from build123d import *

# Parameters (mm, degrees)
SKETCH_1_W                  = 104.137931034
SKETCH_1_H                  = 70
EXTRUDE_1_DEPTH             = 3
SKETCH_2_R                  = 1.75
CUT_EXTRUDE_1_DEPTH         = 10
PATTERN_LINEAR_1_COUNT      = 2
PATTERN_LINEAR_1_PITCH      = 60
PATTERN_LINEAR_1_COUNT_DIR2 = 2
PATTERN_LINEAR_1_PITCH_DIR2 = 40
CUT_EXTRUDE_2_DEPTH         = 4
SKETCH_4_R                  = 4
CUT_EXTRUDE_3_DEPTH         = 4
FILLET_1_R                  = 7


with BuildPart() as part:
    # Эскиз1 → Бобышка-Вытянуть1 (new body)
    with BuildSketch(Plane(origin=(0, 0, 0), x_dir=(1, 0, 0), z_dir=(0, 1, 0))):
        Rectangle(SKETCH_1_W, SKETCH_1_H)
    extrude(amount=EXTRUDE_1_DEPTH)

    # Эскиз2 → Вырез-Вытянуть1 (cut)
    with BuildSketch(Plane(origin=(0, 3, 0), x_dir=(1, 0, 0), z_dir=(0, 1, 0))):
        with Locations((-43.318965517, 26.25)):
            Circle(SKETCH_2_R)
    cut_extrude_1 = extrude(amount=-CUT_EXTRUDE_1_DEPTH, mode=Mode.SUBTRACT)

    # Линейный массив1: Cut-Extrude 1 2 × 2
    with Locations(*[(i * PATTERN_LINEAR_1_PITCH, 0, j * PATTERN_LINEAR_1_PITCH_DIR2) for i in range(PATTERN_LINEAR_1_COUNT) for j in range(PATTERN_LINEAR_1_COUNT_DIR2) if (i, j) != (0, 0)]):
        add(cut_extrude_1, mode=Mode.SUBTRACT)

    # Эскиз3 → Вырез-Вытянуть2 (cut, through all)
    with BuildSketch(Plane(origin=(0, 3, 0), x_dir=(1, 0, 0), z_dir=(0, 1, 0))):
        Polygon((-52.068965517, -22.5), (25.431034483, -22.5), (25.431034483, 35), (52.068965517, 35), (52.068965517, -35), (-52.068965517, -35), align=None)
    extrude(amount=-CUT_EXTRUDE_2_DEPTH, mode=Mode.SUBTRACT)

    # Эскиз4 → Вырез-Вытянуть3 (cut, through all)
    with BuildSketch(Plane(origin=(0, 3, 0), x_dir=(1, 0, 0), z_dir=(0, 1, 0))):
        with Locations((-27.568965517, 6.25)):
            Circle(SKETCH_4_R)
        with BuildLine():
            Line((-13.318965517, 8.5), (8.681034483, 8.5))
            ThreePointArc((8.681034483, 8.5), (10.931034483, 6.25), (8.681034483, 4))
            Line((8.681034483, 4), (-13.318965517, 4))
            ThreePointArc((-13.318965517, 4), (-15.568965517, 6.25), (-13.318965517, 8.5))
        make_face()
    extrude(amount=-CUT_EXTRUDE_3_DEPTH, mode=Mode.SUBTRACT)

    # Скругление1
    fillet_1_edges = [part.edges().sort_by_distance(p)[0] for p in [
        (-52.068965517, 1.5, 22.5),
        (25.431034483, 1.5, 22.5),
        (25.431034483, 1.5, -35),
        (-52.068965517, 1.5, -35),
    ]]
    fillet(fillet_1_edges, radius=FILLET_1_R)


solid = part.part
Work out the finished part from the listing and answer in its coordinate system (mm). A direction names the side the tool comes from. Round coordinates to 2 decimals unless told otherwise and drop trailing zeros. Write each loop counter-clockwise with the first axis right and the second up, starting at its lowest first coordinate (ties: lowest second). Pieces come first, ordered by that corner, then holes. Notation, with made-up numbers: (34, -14.5) -> (73, -14.5) arc R11 ccw to (73, 0.5) -> close; hole circle Ø9 at (60.25, -10). An arc over 180 degrees is marked (long way). Answer as CSV lines item,"result". Start each with the question number.
(1) The part is cut by section D-D, the plane z = -6.25. Give the vertices of the cut face in (x, y), then the cut area to 3 significant figures.
(2) The part is cut by section C-C, the plane y = 0.45. Give the vertices of the cut face in (x, z), then the cut area to 3 significant figures.
(3) Find the intervals of material crossed by probe 1 along X at (y, z) = (1.2, 13.75); probe 2 along X at (y, z) = (1.85, -6.25); probe 3 along Z at (x, y) = (-3, 0.35), in increasing order.
(4) The part is cut by section A-A, the plane z = 13.75. Give the vertices of the cut face in (x, y).
(5) The mould has two halves that part along X. Classify faces 1 (the flat face through (-14, 1, -35)), 2 (the cylindrical face through (15.39, 1.52, -27.43)), 3 (the flat face through (25.431, 2, -6)): +X half, -X half, draft (parallel to the pull), parting line (faces both ways), or undercut.
(6) This flat-tipped pin is pushed along its axis until it touches: pin 1 (2 mm diameter, centred on x = -43.32, z = 13.75, fed in from +Y). Where does it stop, or does it pass through?
(7) The part is cut by section B-B, the plane x = -4.5. Give the vertices of the cut face in (y, z), then the cut area to 3 significant figures.
(8) A tool of negligible diameter and unlimited length cuts with its end or side. For faces 4 (the flat face through (-2, 2, -4)), 5 (the cylindrical face through (23.33, 1.48, 20.5)), from which of +Z, -Z, +X, -X, +Y, -Y can it reach the whole face along a straight path? Write none if from no direction.
Output values:
1,outline,"(-52.07, 0) -> (-31.57, 0) -> (-31.57, 3) -> (-52.07, 3) -> close; (-23.57, 0) -> (-15.57, 0) -> (-15.57, 3) -> (-23.57, 3) -> close; (10.93, 0) -> (25.43, 0) -> (25.43, 3) -> (10.93, 3) -> close"
1,area,"129 mm²"
2,outline,"(-52.07, -28) arc R7 ccw to (-45.07, -35) -> (18.43, -35) arc R7 ccw to (25.43, -28) -> (25.43, 15.5) arc R7 ccw to (18.43, 22.5) -> (-45.07, 22.5) arc R7 ccw to (-52.07, 15.5) -> close; hole circle Ø3.5 at (-43.32, -26.25); hole circle Ø3.5 at (-43.32, 13.75); hole circle Ø8 at (-27.57, -6.25); hole (-13.32, -8.5) -> (8.68, -8.5) arc R2.25 ccw to (8.68, -4) -> (-13.32, -4) arc R2.25 ccw to start; hole circle Ø3.5 at (16.68, -26.25); hole circle Ø3.5 at (16.68, 13.75)"
2,area,"4,210 mm²"
3,probe 1,"x = -52.07 to -45.07, -41.57 to 14.93, 18.43 to 25.43"
3,probe 2,"x = -52.07 to -31.57, -23.57 to -15.57, 10.93 to 25.43"
3,probe 3,"z = -35 to -8.5, -4 to 22.5"
4,outline,"(-52.07, 0) -> (-45.07, 0) -> (-45.07, 3) -> (-52.07, 3) -> close; (-41.57, 0) -> (14.93, 0) -> (14.93, 3) -> (-41.57, 3) -> close; (18.43, 0) -> (25.43, 0) -> (25.43, 3) -> (18.43, 3) -> close"
5,face 1,"draft"
5,face 2,"undercut"
5,face 3,"+X half"
6,pin 1,"passes through"
7,outline,"(0, -35) -> (3, -35) -> (3, -8.5) -> (0, -8.5) -> close; (0, -4) -> (3, -4) -> (3, 22.5) -> (0, 22.5) -> close"
7,area,"159 mm²"
8,face 4,"+Y, -Y"
8,face 5,"+Z, +X, +Y, -Y"
